Model file for the job. Use its own axes, mm. A direction names the side the tool comes from. Coordinates: 2 decimals unless noted, no trailing zeros. Write each loop counter-clockwise with the first axis right and the second up, starting at its lowest first coordinate (ties: lowest second). Pieces come first, ordered by that corner, then holes.
Q1. Band-saw the part on D-D, the plane z = 2. Write the cut outline in (x, y).
Q2. Band-saw the part on C-C, the plane z = 10. Write the cut outline in (x, y).
Q3. Drill centre lines: probe 1 along Y at (x, z) = (0, 11.75); probe 2 along Y at (x, z) = (0, 9); probe 3 along X at (y, z) = (-18.5, 11.25). Where is each one in solid material? Low to high.
Q4. Band-saw the part on A-A, the plane y = 0. Write the cut outline in (x, z).
Q5. Which spindle directions (+Z, -Z, +X, -X, +Y, -Y) get a long thin tool onto all of the face, cutting with end or side? Do faces 1 (the flat face through (0, 0, 6.35)), 2 (the flat face through (0, 0, 0)). Say none if no direction does.
Q6. Pin check, flat tips, straight feed: P1, Ø4, axis at y = -4.5, z = 10, coming from the +X side; P2, Ø8, axis at x = 0, y = 0, coming from the +Z side; P3, Ø2, axis at x = 12.5, z = 11, coming from the +Y side; P4, Ø6, axis at y = -8.5, z = 6.5, coming from the +X side. Stop position of each tip, or through.
from build123d import *

# Parameters (mm, degrees)
F0_R     = 38.1
F1_DEPTH = 12.7
F2_R     = 5.08
F3_R     = 3.429
F4_DEPTH = 6.35


with BuildPart() as f1:
    # F0 (on Top) → F1 (new body)
    with BuildSketch(Plane.XY):
        Circle(F0_R)
    extrude(amount=F1_DEPTH)

    # F2
    f2_edges = [f1.edges().sort_by_distance(p)[0] for p in [
        (-38.1, 0, 0),
        (-38.1, 0, 12.7),
    ]]
    fillet(f2_edges, radius=F2_R)

    # F3 (on face) → F4 (cut)
    with BuildSketch(Plane.XY.offset(12.7)):
        Circle(F3_R)
    extrude(amount=-F4_DEPTH, mode=Mode.SUBTRACT)


solid = f1.part
Answer sheet:
1. outline: circle Ø74.12 at (0, 0)
2. outline: circle Ø75.02 at (0, 0); hole circle Ø6.86 at (0, 0)
3. probe 1: y = -35.98 to -3.43, 3.43 to 35.98
3. probe 2: y = -37.91 to -3.43, 3.43 to 37.91
3. probe 3: x = -31.55 to 31.55
4. outline: (-38.1, 5.08) arc R5.08 ccw to (-33.02, 0) - (33.02, 0) arc R5.08 ccw to (38.1, 5.08) - (38.1, 7.62) arc R5.08 ccw to (33.02, 12.7) - (3.43, 12.7) - (3.43, 6.35) - (-3.43, 6.35) - (-3.43, 12.7) - (-33.02, 12.7) arc R5.08 ccw to (-38.1, 7.62) - close
5. face 1: +Z
5. face 2: -Z, +X, -X, +Y, -Y
6. P1: stops at x = 37.9
6. P2: stops at z = 12.7
6. P3: stops at y = 35.46
6. P4: stops at x = 37.7
